Verification items for the finished model (mm, model axes). Face numbers are marked on the shaded views. Coordinates: 2 decimals unless noted, no trailing zeros. Write each loop counter-clockwise with the first axis right and the second up, starting at its lowest first coordinate (ties: lowest second). Pieces come first, ordered by that corner, then holes. Notation, with made-up numbers: (8.5, -37.75) -> (14.5, -37.75) arc R18 cw to (14.5, -28.75) -> close; hole circle Ø3 at (-10.75, -22.75). An arc over 180 degrees is marked (long way). Answer in a Markdown table with one row per item.
```python
from build123d import *

# Parameters (mm, degrees)
F0_W        = 40
F0_H        = 24
F0_R        = 2.5
F0_R_2      = 7.5
F1_DEPTH    = 4
F3_DEPTH    = 81
F4_D        = 5.5
F4_DEPTH    = 4
F4_TIP      = 1.6523667023
F6_DEPTH    = 75
F7_T2_ANGLE = 287.359476763
F7_T4_ANGLE = 107.2329087186
F8_R        = 7.5
F9_DEPTH    = 2
F10_R       = 1


# Not quite as in the source:
# - a fillet or chamfer that OpenCascade refuses, or shapes differently, is made with other operations: its cross-section is extruded or revolved along the edge and cut away or added


with BuildPart() as f1:
    # F0 (on Front) → F1 (new body)
    with BuildSketch(Plane.XZ):
        with Locations((20, 12)):
            Rectangle(F0_W, F0_H)
        with Locations((7, 12)):
            Circle(F0_R, mode=Mode.SUBTRACT)
        with Locations((20, 12)):
            Circle(F0_R_2, mode=Mode.SUBTRACT)
        with Locations((33, 12)):
            Circle(F0_R, mode=Mode.SUBTRACT)
        with Locations((20, 12)):
            Circle(F0_R_2)
        with Locations((7, 12)):
            Circle(F0_R)
        with Locations((33, 12)):
            Circle(F0_R)
    extrude(amount=-F1_DEPTH)

    # F0 (on Front) → F3 (join)
    with BuildSketch(Plane.XZ):
        with Locations((20, 12)):
            Circle(F0_R_2)
    extrude(amount=F3_DEPTH)

    # F4
    with Locations(Plane.XZ):
        with Locations((33, 12), (7, 12)):
            Hole(F4_D / 2, depth=F4_DEPTH)
            with Locations((0, 0, -(F4_DEPTH + F4_TIP / 2))):  # 118° drill point
                Cone(0, F4_D / 2, F4_TIP, mode=Mode.SUBTRACT)

    # F5 (on face) → F6 (cut)
    with BuildSketch(Plane.XZ.offset(81)):
        with BuildLine():
            ThreePointArc((23.7416573868, 18.5), (20, 19.5), (16.2583426132, 18.5))
            Line((16.2583426132, 18.5), (23.7416573868, 18.5))
        make_face()
    extrude(amount=-F6_DEPTH, mode=Mode.SUBTRACT)

    # F7: chamfer of 1 on 2 edges, made by hand

    # F7_s1 → F7_t2 (revolve, cut)
    with BuildSketch(Plane(origin=(14.8022480235, 0, -4.6272486525), x_dir=(0, 1, 0), z_dir=(0.9544515906, 0, -0.2983658178))):
        with BuildLine():
            Line((-79.9717157288, 24.9490197138), (-81.0282842712, 23.8924511713))
            Line((-81.0282842712, 23.8924511713), (-81.0482842712, 23.8924511713))
            ThreePointArc((-81.0482842712, 23.8924511713), (-81.02, 24.406593307), (-81.02, 24.9207354426))
            Line((-81.02, 24.9207354426), (-81, 24.9407354426))
            ThreePointArc((-81, 24.9407354426), (-80.4858578644, 24.9407354426), (-79.9717157288, 24.9690197138))
            Line((-79.9717157288, 24.9690197138), (-79.9717157288, 24.9490197138))
        make_face()
    revolve(axis=Axis((20, -81, 12), (0, -1, 0)), revolution_arc=F7_T2_ANGLE, mode=Mode.SUBTRACT)

    # F7_s3 → F7_t4 (revolve, cut)
    with BuildSketch(Plane.XY.offset(12)):
        with BuildLine():
            Line((27.5282842712, -79.9717157288), (26.4717157288, -81.0282842712))
            Line((26.4717157288, -81.0282842712), (26.4717157288, -81.0482842712))
            ThreePointArc((26.4717157288, -81.0482842712), (26.9858578644, -81.02), (27.5, -81.02))
            Line((27.5, -81.02), (27.52, -81))
            ThreePointArc((27.52, -81), (27.52, -80.4858578644), (27.5482842712, -79.9717157288))
            Line((27.5482842712, -79.9717157288), (27.5282842712, -79.9717157288))
        make_face()
    revolve(axis=Axis((20, -81, 12), (0, -1, 0)), revolution_arc=F7_T4_ANGLE, mode=Mode.SUBTRACT)

    # F8 (on face) → F9 (cut)
    with BuildSketch(Plane(origin=(0, 4, 0), x_dir=(-1, 0, 0), z_dir=(0, 1, 0))):
        with Locations((-20, 12)):
            Circle(F8_R)
    extrude(amount=-F9_DEPTH, mode=Mode.SUBTRACT)

    # F10
    f10_edges = [f1.edges().sort_by_distance(p)[0] for p in [
        (0, 2, 24),
        (0, 2, 0),
        (40, 2, 0),
        (40, 2, 24),
        (27.5, 2, 12),
    ]]
    fillet(f10_edges, radius=F10_R)


solid = f1.part
```
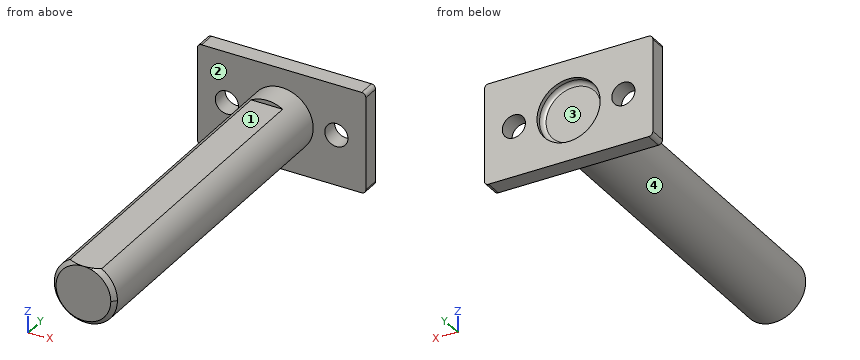
1. Sectioned sample at C-C, the plane x = 37. Record the cut outline in (y, z), and give its area (3 significant figures).
Findings below:
| item | result |
|---|---|
| outline | (0, 0) -> (4, 0) -> (4, 24) -> (0, 24) -> close |
| area | 96.0 mm² |
2. Go/stop test with flat-tipped pins: pin 1 (1.1 mm diameter, centred on x = 19.5, z = 19, fed in from -Y); pin 2 (4 mm diameter, centred on x = 21.5, z = 9, fed in from +Y); pin 3 (5 mm diameter, centred on x = 7, z = 12, fed in from -Y); pin 4 (3 mm diameter, centred on y = -13, z = 18, fed in from +X). Record where each tip stops, or that it passes through.
Findings below:
| item | result |
|---|---|
| pin 1 | stops at y = -81 |
| pin 2 | stops at y = 2 |
| pin 3 | passes through |
| pin 4 | stops at x = 26 |
3. Material ranges on probe 1 along Z at (x, y) = (7, 1.6); probe 2 along X at (y, z) = (-8.5, 5.5); probe 3 along Y at (x, z) = (20, 7), recorded low to high. Write a range as from..to.
Findings below:
| item | result |
|---|---|
| probe 1 | z = 0..9.25, 14.75..24 |
| probe 2 | x = 16.26..23.74 |
| probe 3 | y = -81..2 |
4. Sectioned sample at B-B, the plane y = -47. Record the cut outline in (x, z).
Findings below:
| item | result |
|---|---|
| outline | (16.26, 18.5) arc R7.5 ccw (long way) to (23.74, 18.5) -> close |
5. Release check for a two-part mould opening along Z. For the marked faces 1, 2, 3 and 4 record: released by +Z, released by -Z, zero draft, split by the parting line, or undercut.
Findings below:
| item | result |
|---|---|
| face 1 | released by +Z |
| face 2 | zero draft |
| face 3 | undercut |
| face 4 | split by the parting line |
6. Sectioned sample at A-A, the plane x = 7. Record the cut outline in (y, z), and give its area (3 significant figures).
Findings below:
| item | result |
|---|---|
| outline | (0, 0) -> (4, 0) -> (4, 9.25) -> (0, 9.25) -> close; (0, 14.75) -> (4, 14.75) -> (4, 24) -> (0, 24) -> close |
| area | 74.0 mm² |
